Geometry: final body of the model. Coordinates: model frame, mm. Coordinates: 2 decimals unless noted, no trailing zeros. Use one line per item in the form item = value.
```python
from build123d import *

# Parameters (mm, degrees)
SKETCH1_W           = 500
SKETCH1_H           = 30
BOSS_EXTRUDE1_DEPTH = 6.35
SKETCH2_R           = 3.175
CUT_EXTRUDE1_DEPTH  = 3
CUT_EXTRUDE2_DEPTH  = 402.147008589
SKETCH6_R           = 1.89865
CUT_EXTRUDE3_DEPTH  = 404.162898219


with BuildPart() as part:
    # Sketch1 → Boss-Extrude1 (new body)
    with BuildSketch(Plane(origin=(0, 2, 0), x_dir=(-1, 0, 0), z_dir=(0, -1, 0))):
        with Locations((-150, 35)):
            Rectangle(SKETCH1_W, SKETCH1_H)
    extrude(amount=BOSS_EXTRUDE1_DEPTH)

    # Sketch2 → Cut-Extrude1 (cut)
    with BuildSketch(Plane.XZ.offset(-2)):
        with Locations((5, -28)):
            Circle(SKETCH2_R)
        with Locations((-66.5, -42)):
            Circle(SKETCH2_R)
        with Locations((-66.5, -28)):
            Circle(SKETCH2_R)
        with Locations((5, -42)):
            Circle(SKETCH2_R)
        with Locations((76.5, -28)):
            Circle(SKETCH2_R)
        with Locations((76.5, -42)):
            Circle(SKETCH2_R)
        with Locations((148, -28)):
            Circle(SKETCH2_R)
        with Locations((148, -42)):
            Circle(SKETCH2_R)
        with Locations((219.5, -28)):
            Circle(SKETCH2_R)
        with Locations((219.5, -42)):
            Circle(SKETCH2_R)
        with Locations((291, -28)):
            Circle(SKETCH2_R)
        with Locations((291, -42)):
            Circle(SKETCH2_R)
        with Locations((362.5, -28)):
            Circle(SKETCH2_R)
        with Locations((362.5, -42)):
            Circle(SKETCH2_R)
    extrude(amount=CUT_EXTRUDE1_DEPTH, mode=Mode.SUBTRACT)

    # Sketch5 → Cut-Extrude2 (cut, through all)
    with BuildSketch(Plane(origin=(0, 0, -50), x_dir=(-1, 0, 0), z_dir=(0, 0, -1))):
        Polygon((-1.574705718, 2.00006084), (-0.057166038, 2.00006084), (-0.057166038, -0.05708916), (1.644633962, -0.05708916), (1.644633962, 2.00006084), (15.542833962, 2.00006084), (15.542833962, -0.05708916), (17.244633962, -0.05708916), (17.244633962, 2.00006084), (23.142833962, 2.00006084), (23.142833962, -0.05708916), (24.844633962, -0.05708916), (24.844633962, 2.00006084), (33.742833962, 2.00006084), (33.742833962, -0.05708916), (35.444633962, -0.05708916), (35.444633962, 2.00006084), (44.342833962, 2.00006084), (44.342833962, -0.05708916), (46.044633962, -0.05708916), (46.044633962, 2.00006084), (54.942833962, 2.00006084), (54.942833962, -0.05708916), (56.644633962, -0.05708916), (56.644633962, 2.00006084), (61.710485811, 2.00006084), (61.710485811, 3.366834616), (-1.574705718, 3.366834616), align=None)
        Polygon((-73.074705718, 2.00006084), (-71.557166038, 2.00006084), (-71.557166038, -0.05708916), (-69.855366038, -0.05708916), (-69.855366038, 2.00006084), (-55.957166038, 2.00006084), (-55.957166038, -0.05708916), (-54.255366038, -0.05708916), (-54.255366038, 2.00006084), (-48.357166038, 2.00006084), (-48.357166038, -0.05708916), (-46.655366038, -0.05708916), (-46.655366038, 2.00006084), (-37.757166038, 2.00006084), (-37.757166038, -0.05708916), (-36.055366038, -0.05708916), (-36.055366038, 2.00006084), (-27.157166038, 2.00006084), (-27.157166038, -0.05708916), (-25.455366038, -0.05708916), (-25.455366038, 2.00006084), (-16.557166038, 2.00006084), (-16.557166038, -0.05708916), (-14.855366038, -0.05708916), (-14.855366038, 2.00006084), (-9.789514189, 2.00006084), (-9.789514189, 3.366834616), (-73.074705718, 3.366834616), align=None)
        Polygon((-144.574705718, 2.00006084), (-143.057166038, 2.00006084), (-143.057166038, -0.05708916), (-141.355366038, -0.05708916), (-141.355366038, 2.00006084), (-127.457166038, 2.00006084), (-127.457166038, -0.05708916), (-125.755366038, -0.05708916), (-125.755366038, 2.00006084), (-119.857166038, 2.00006084), (-119.857166038, -0.05708916), (-118.155366038, -0.05708916), (-118.155366038, 2.00006084), (-109.257166038, 2.00006084), (-109.257166038, -0.05708916), (-107.555366038, -0.05708916), (-107.555366038, 2.00006084), (-98.657166038, 2.00006084), (-98.657166038, -0.05708916), (-96.955366038, -0.05708916), (-96.955366038, 2.00006084), (-88.057166038, 2.00006084), (-88.057166038, -0.05708916), (-86.355366038, -0.05708916), (-86.355366038, 2.00006084), (-81.289514189, 2.00006084), (-81.289514189, 3.366834616), (-144.574705718, 3.366834616), align=None)
        Polygon((-216.074705718, 2.00006084), (-214.557166038, 2.00006084), (-214.557166038, -0.05708916), (-212.855366038, -0.05708916), (-212.855366038, 2.00006084), (-198.957166038, 2.00006084), (-198.957166038, -0.05708916), (-197.255366038, -0.05708916), (-197.255366038, 2.00006084), (-191.357166038, 2.00006084), (-191.357166038, -0.05708916), (-189.655366038, -0.05708916), (-189.655366038, 2.00006084), (-180.757166038, 2.00006084), (-180.757166038, -0.05708916), (-179.055366038, -0.05708916), (-179.055366038, 2.00006084), (-170.157166038, 2.00006084), (-170.157166038, -0.05708916), (-168.455366038, -0.05708916), (-168.455366038, 2.00006084), (-159.557166038, 2.00006084), (-159.557166038, -0.05708916), (-157.855366038, -0.05708916), (-157.855366038, 2.00006084), (-152.789514189, 2.00006084), (-152.789514189, 3.366834616), (-216.074705718, 3.366834616), align=None)
        Polygon((-287.574705718, 2.00006084), (-286.057166038, 2.00006084), (-286.057166038, -0.05708916), (-284.355366038, -0.05708916), (-284.355366038, 2.00006084), (-270.457166038, 2.00006084), (-270.457166038, -0.05708916), (-268.755366038, -0.05708916), (-268.755366038, 2.00006084), (-262.857166038, 2.00006084), (-262.857166038, -0.05708916), (-261.155366038, -0.05708916), (-261.155366038, 2.00006084), (-252.257166038, 2.00006084), (-252.257166038, -0.05708916), (-250.555366038, -0.05708916), (-250.555366038, 2.00006084), (-241.657166038, 2.00006084), (-241.657166038, -0.05708916), (-239.955366038, -0.05708916), (-239.955366038, 2.00006084), (-231.057166038, 2.00006084), (-231.057166038, -0.05708916), (-229.355366038, -0.05708916), (-229.355366038, 2.00006084), (-224.289514189, 2.00006084), (-224.289514189, 3.366834616), (-287.574705718, 3.366834616), align=None)
        Polygon((-359.074705718, 2.00006084), (-357.557166038, 2.00006084), (-357.557166038, -0.05708916), (-355.855366038, -0.05708916), (-355.855366038, 2.00006084), (-341.957166038, 2.00006084), (-341.957166038, -0.05708916), (-340.255366038, -0.05708916), (-340.255366038, 2.00006084), (-334.357166038, 2.00006084), (-334.357166038, -0.05708916), (-332.655366038, -0.05708916), (-332.655366038, 2.00006084), (-323.757166038, 2.00006084), (-323.757166038, -0.05708916), (-322.055366038, -0.05708916), (-322.055366038, 2.00006084), (-313.157166038, 2.00006084), (-313.157166038, -0.05708916), (-311.455366038, -0.05708916), (-311.455366038, 2.00006084), (-302.557166038, 2.00006084), (-302.557166038, -0.05708916), (-300.855366038, -0.05708916), (-300.855366038, 2.00006084), (-295.789514189, 2.00006084), (-295.789514189, 3.366834616), (-359.074705718, 3.366834616), align=None)
    extrude(amount=-CUT_EXTRUDE2_DEPTH, mode=Mode.SUBTRACT)

    # Sketch6 → Cut-Extrude3 (cut, through all)
    with BuildSketch(Plane.XZ.offset(4.35)):
        with Locations((-66.5, -42)):
            Circle(SKETCH6_R)
        with Locations((-66.5, -28)):
            Circle(SKETCH6_R)
        with Locations((5, -42)):
            Circle(SKETCH6_R)
        with Locations((5, -28)):
            Circle(SKETCH6_R)
        with Locations((76.5, -42)):
            Circle(SKETCH6_R)
        with Locations((76.5, -28)):
            Circle(SKETCH6_R)
        with Locations((148, -42)):
            Circle(SKETCH6_R)
        with Locations((148, -28)):
            Circle(SKETCH6_R)
        with Locations((219.5, -42)):
            Circle(SKETCH6_R)
        with Locations((219.5, -28)):
            Circle(SKETCH6_R)
        with Locations((291, -42)):
            Circle(SKETCH6_R)
        with Locations((291, -28)):
            Circle(SKETCH6_R)
        with Locations((362.5, -42)):
            Circle(SKETCH6_R)
        with Locations((362.5, -28)):
            Circle(SKETCH6_R)
    extrude(amount=-CUT_EXTRUDE3_DEPTH, mode=Mode.SUBTRACT)


solid = part.part
```
1) Material intervals for probe 1 along Z at (x, y) = (148, -2.15); probe 2 along Z at (x, y) = (219.5, 1.35) (3 decimals); probe 3 along Y at (x, z) = (-23.5, -42.75), sorted ascending. Write a range as from..to.
Results found:
probe_1 = -50..-43.9, -40.1..-29.9, -26.1..-20
probe_2 = -50..-45.175, -38.825..-31.175, -24.825..-20
probe_3 = -4.35..-0.06
2) Contact query for a flat-ended pin moving along its axis: P1, Ø0.5, axis at x = 333, z = -39.5, coming from the +Y side. Output: stop coordinate, or through.
Results found:
P1 = -0.06
3) Section A-A, the plane y = 1. Give the number of separate pieces and of enclosed holes in the cut face, and give its area (3 significant figures).
Results found:
separate_pieces = 37
enclosed_holes = 14
area = 12,700 mm2
